Autodesk Inventor part; units mm, degrees
ref_plane "YZ Plane" through (0, 0, 0) normal (1, 0, 0) x (0, 1, 0)
ref_plane "XZ Plane" through (0, 0, 0) normal (0, 1, 0) x (-1, 0, 0)
ref_plane "XY Plane" through (0, 0, 0) normal (0, 0, 1) x (1, 0, 0)
sketch "Sketch1" plane through (0, 0, 0) normal (0, 0, 1) x (1, 0, 0)
  line L0 (0, 7.7456) -> (30, 7.7456)
  line L1 (30, 7.7456) -> (32, -2.2544)
  line L2 (32, -2.2544) -> (73, -2.2544)
  line L3 (73, -2.2544) -> (75, 7.7456)
  line L4 (23, -17.2544) -> (25, -17.2544)
  line L5 (25, -17.2544) -> (25, 2.7456)
  line L6 (25, 2.7456) -> (6, 2.7456)
  line L7 (75, 7.7456) -> (80, 7.7456)
  line L8 (80, 7.7456) -> (80, -5.2544)
  line L9 (80, -5.2544) -> (25, -22.2544)
  line L10 (25, -22.2544) -> (23, -17.2544)
  line L11 (0, 7.7456) -> (0, 2.7456)
  line L12 (0, 2.7456) -> (6, 2.7456)
  point P0 (0, 0)
  dimension "d0" = 20
  dimension "d4" = 5
  dimension "d7" = 2
  dimension "d8" = 10
  dimension "d9" = 45
  dimension "d11" = 41
  dimension "d12" = 2
  dimension "d13" = 5
  dimension "d14" = 13
  dimension "d15" = 5
  dimension "d18" = 0
  dimension "d19" = 6
  dimension "d20" = 30
  dimension "d21" = 25
  dimension "d26" = 2.7456
  dimension "d27" = 2.7456
extrude "Extrusion1" add sketch "Sketch1" along normal mid plane 18
sketch "Sketch4" plane through (0, 2.7456, 9) normal (0, -1, 0) x (1, 0, 0)
  arc A0 (-1.1431, -18) -> (-1.1431, 0) centre (-36, -9) ccw
  line L0 (0, 0) -> (0, -18)
  arc A1 (5.0244, -18) -> (5.0244, 0) centre (-36, -9) ccw
  arc A2 (-4.251, -18) -> (-4.251, 0) centre (-36, -9) ccw
  line L1 (30, 0) -> (0, 0)
  line L2 (5.0244, 0) -> (-4.251, 0)
  line L3 (0, -18) -> (30, -18)
  line L4 (5.0244, -18) -> (-4.251, -18)
  point P0 (0, -9)
  dimension "d28" = 72
  dimension "d29" = 36
  dimension "d30" = 84
  dimension "d31" = 66
extrude "Extrusion2" add sketch "Sketch4" against normal blind 5
extrude "Extrusion3" add sketch "Sketch4" along normal blind 3 contours L4 A2 L2 A0
extrude "Extrusion4" cut sketch "Sketch4" against normal blind 2 contours A0 L0 L4 | A0 L2 L0 | L0 L1 A1 L3
fillet "Fillet1" radius 2 2 edges at (30, 7.7456, 0) (75, 7.7456, 0)
fillet "Fillet2" radius 2 5 edges at (73, -2.2544, 0) (32, -2.2544, 0) (25, -22.2544, 0) (80, -5.2544, 0) (80, 7.7456, 0)
fillet "Fillet3" radius 1 2 edges at (-3, 7.7456, 0) (-3, -0.2544, 0)
sketch "Sketch5" plane through (0, 0, 9) normal (0, 0, 1) x (1, 0, 0)
  line L0 (30, -6.7544) -> (60.4607, -6.7544)
  line L1 (60.4607, -6.7544) -> (30, -16.6287)
  line L2 (30, -16.6287) -> (30, -6.7544)
  line L3 (71.3604, -2.2544) -> (33.6396, -2.2544)
  line L4 (26.7625, -21.7097) -> (78.5906, -5.6901)
  line L5 (25, 2.7456) -> (25, -17.2544)
  point P0 (0, 0)
  dimension "d41" = 4.5
  dimension "d42" = 0.785
  dimension "d43" = 5
extrude "Extrusion5" cut sketch "Sketch5" against normal through all
fillet "Fillet4" radius 1 3 edges at (60.4607, -6.7544, 0) (30, -6.7544, 0) (30, -16.6287, 0)
equation "\"d29\" = 0.5 * d28"
properties part number "HeadphoneMount"
Check sheet for the modelled part. Datum: model origin and axes. Units: mm. A direction names the side the tool comes from. Round coordinates to 2 decimals unless told otherwise and drop trailing zeros. Write each loop counter-clockwise with the first axis right and the second up, starting at its lowest first coordinate (ties: lowest second). Pieces come first, ordered by that corner, then holes. Notation, with made-up numbers: M -34,64 L 21,64 A26 cw 21,89 Z; hole C 87,4 d3. An arc over 180 degrees is marked long. Write item = value, one per line. Start each with the question number.
1. Scan lines: line 1 (X direction, y = 0.25, z = 7); line 2 (X direction, y = 1.5, z = 6.5); line 3 (Y direction, x = 15.5, z = -6). Record each from-to range of solid material in increasing order. Write a range as [from, to].
2. Section check C-C, the plane x = 14.5. Record the cut outline in (y, z), then the cut area to 3 significant figures.
3. Tool access check on faces 1 (the flat face through (42, -6.754, 0)), 2 (the flat face through (-1, -0.254, 0)), 3 (the cylindrical face through (72.64, -1.79, -0.13)), 4 (the flat face through (24, -17.254, 0)), 5 (the cylindrical face through (79.62, -4.95, -0.13)). Record the directions out of +Z, -Z, +X, -X, +Y, -Y that give a thin tool (end or side, any length) a straight path to the whole face; none if there is none.
4. Section check D-D, the plane y = -18. Record the cut outline in (x, z), then the cut area to 3 significant figures.
5. Section check A-A, the plane x = 42. Record the cut outline in (y, z).
6. Section check B-B, the plane y = -1.5. Record the cut outline in (x, z).
7. Release check for a two-part mould opening along Z. For faces 6 (the flat face through (41, -3, -9)), 7 (the flat face through (53, -13.6, -0.1)), 8 (the cylindrical face through (0, 2, 0)), 9 (the cylindrical face through (-3, 4, 0)) record: pulls with the +Z half, pulls with the -Z half, needs draft (parallel to the pull), parting line crosses it, or undercut.
8. Gauge pin test, flat ends, axial feed: pin 1 (2 mm diameter, centred on x = 1.5, z = 3.5, fed in from -Y); pin 2 (9 mm diameter, centred on y = -9.5, z = 3.5, fed in from -X); pin 3 (8 mm diameter, centred on x = 33.5, z = 7, fed in from +Y). Record the tip position at first contact, or that the pin passes through.
Results found:
q1.line_1 = [-3.62, -0.69], [25, 31.5], [73.5, 80]
q1.line_2 = [-3.65, -0.59], [25, 31.25], [73.75, 80]
q1.line_3 = [2.75, 7.75]
q2.outline = M 2.75,-9 L 7.75,-9 L 7.75,9 L 2.75,9 Z
q2.area = 90.0 mm^2
q3.face_1 = +Z, -Z
q3.face_2 = +Z, -Z, -X, -Y
q3.face_3 = +Z, -Z, +Y
q3.face_4 = +Z, -Z, -X
q3.face_5 = +Z, -Z, +X, -Y
q4.outline = M 23.3,-9 L 38.76,-9 L 38.76,9 L 23.3,9 Z
q4.area = 278 mm^2
q5.outline = M -17,-9 L -12.74,-9 L -12.74,9 L -17,9 Z; M -6.75,-9 L -2.25,-9 L -2.25,9 L -6.75,9 Z
q6.outline = M 25,-9 L 32.07,-9 L 32.07,9 L 25,9 Z; M 72.93,-9 L 80,-9 L 80,9 L 72.93,9 Z
q7.face_6 = pulls with the -Z half
q7.face_7 = needs draft
q7.face_8 = parting line crosses it
q7.face_9 = undercut
q8.pin_1 = 4.75
q8.pin_2 = 25
q8.pin_3 = 7.39
